The model under review builds one solid part; all positions refer to its coordinate system, in mm. Coordinates: 2 decimals unless noted, no trailing zeros. Write each loop counter-clockwise with the first axis right and the second up, starting at its lowest first coordinate (ties: lowest second). Pieces come first, ordered by that corner, then holes. Notation, with made-up numbers: M -25.5,-39.5 L 27.5,-39.5 A23 cw 27.5,-8.5 Z; hole C -31,74 d8. An arc over 180 degrees is marked long. Answer as a JSON object with one key per item and string values.
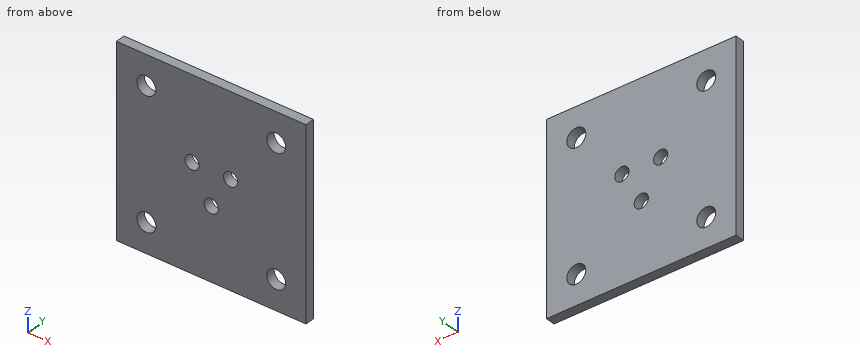
```python
from build123d import *

# Parameters (mm, degrees)
SKETCH1_W           = 63.5
SKETCH1_H           = 63.5
BOSS_EXTRUDE1_DEPTH = 3.175
SKETCH2_R           = 2.38125
CUT_EXTRUDE1_DEPTH  = 4.175
SKETCH3_R           = 3.175
CUT_EXTRUDE2_DEPTH  = 4.175


with BuildPart() as part:
    # Sketch1 → Boss-Extrude1 (new body)
    with BuildSketch(Plane(origin=(0, 0, 0), x_dir=(1, 0, 0), z_dir=(0, 1, 0))):
        Rectangle(SKETCH1_W, SKETCH1_H)
    extrude(amount=BOSS_EXTRUDE1_DEPTH)

    # Sketch2 → Cut-Extrude1 (cut, through all)
    with BuildSketch(Plane(origin=(0, 3.175, 0), x_dir=(1, 0, 0), z_dir=(0, 1, 0))):
        with Locations((0, 7.5)):
            Circle(SKETCH2_R)
        with Locations((6.495190528, -3.75)):
            Circle(SKETCH2_R)
        with Locations((-6.495190528, -3.75)):
            Circle(SKETCH2_R)
    extrude(amount=-CUT_EXTRUDE1_DEPTH, mode=Mode.SUBTRACT)

    # Sketch3 → Cut-Extrude2 (cut, through all)
    with BuildSketch(Plane(origin=(0, 3.175, 0), x_dir=(1, 0, 0), z_dir=(0, 1, 0))):
        with Locations((-21.75, 21.75)):
            Circle(SKETCH3_R)
        with Locations((-21.75, -21.75)):
            Circle(SKETCH3_R)
        with Locations((21.75, -21.75)):
            Circle(SKETCH3_R)
        with Locations((21.75, 21.75)):
            Circle(SKETCH3_R)
    extrude(amount=-CUT_EXTRUDE2_DEPTH, mode=Mode.SUBTRACT)


solid = part.part
```
(1) Add section C-C on y = 1.85. Count the separate pieces of the cut face and the enclosed holes in it, and give its area (3 significant figures).
Results list:
{"separate pieces": "1", "enclosed holes": "7", "area": "3,850 mm²"}
(2) Add section A-A on z = -7.5. Give the boundary of the cut face in (x, y) (3 decimals).
Results list:
{"outline": "M -31.75,0 L -2.381,0 L -2.381,3.175 L -31.75,3.175 Z; M 2.381,0 L 31.75,0 L 31.75,3.175 L 2.381,3.175 Z"}
(3) Wall thickness on line 1 along Z through (x, y) = (21.75, 1.05) (3 decimals); line 2 along X through (y, z) = (1.35, 3.75): over which ranges is each line inside the solid? List them lowest first. Write a range as from..to.
Results list:
{"line 1": "-31.75..-24.925, -18.575..18.575, 24.925..31.75", "line 2": "-31.75..-8.88, -4.11..4.11, 8.88..31.75"}
(4) Add section B-B on x = 0. Give the boundary of the cut face in (y, z) (3 decimals), and give its area (3 significant figures).
Results list:
{"outline": "M 0,-31.75 L 3.175,-31.75 L 3.175,-9.881 L 0,-9.881 Z; M 0,-5.119 L 3.175,-5.119 L 3.175,31.75 L 0,31.75 Z", "area": "186 mm²"}
(5) Add section D-D on x = 21.75. Give the boundary of the cut face in (y, z) (3 decimals).
Results list:
{"outline": "M 0,-31.75 L 3.175,-31.75 L 3.175,-24.925 L 0,-24.925 Z; M 0,-18.575 L 3.175,-18.575 L 3.175,18.575 L 0,18.575 Z; M 0,24.925 L 3.175,24.925 L 3.175,31.75 L 0,31.75 Z"}
